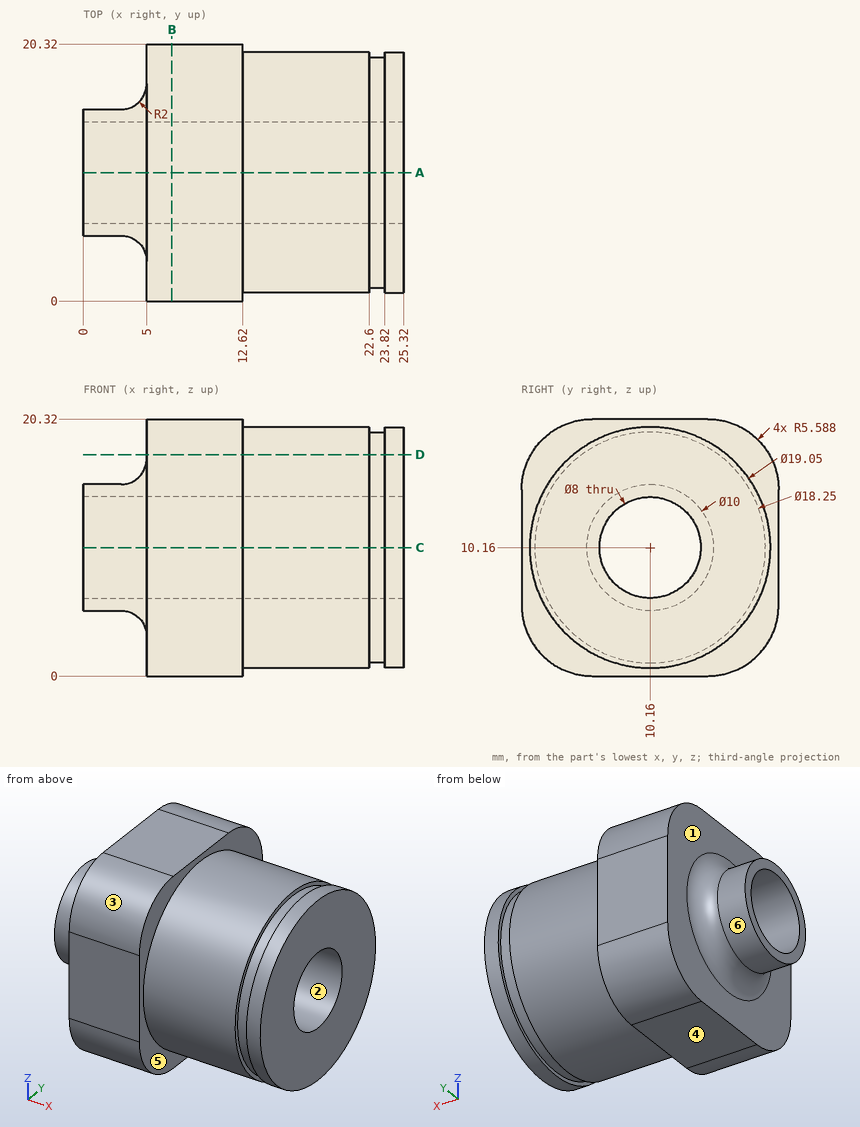
The drawing under review shows one solid part. Ordinate dimensions are in mm from its lowest x, y, z. A direction names the side the tool comes from. Coordinates: 2 decimals unless noted, no trailing zeros. Loops run counter-clockwise (first coordinate to the right, second up) from the corner with the lowest first, then second, coordinate; pieces in that order, holes last. Notation, with made-up numbers: (85.5, 39) - (97.5, 39) arc R27 ccw to (97.5, 65) - close; hole circle Ø5 at (27, -36.5). An arc over 180 degrees is marked (long way). Return JSON: item names as keys, results as strings.
Item 1: Take a section at B-B (x = 7). Give the boundary of the cut face in (y, z), then the cut area to 3 significant figures.
Determined:
{"outline": "(0, 5.59) arc R5.59 ccw to (5.59, 0) - (14.73, 0) arc R5.59 ccw to (20.32, 5.59) - (20.32, 14.73) arc R5.59 ccw to (14.73, 20.32) - (5.59, 20.32) arc R5.59 ccw to (0, 14.73) - close; hole circle Ø8 at (10.16, 10.16)", "area": "336 mm2"}
Item 2: For the marked faces 4, 5 and 6, list the 3-axis set-ups (+Z, -Z, +X, -X, +Y, -Y) from which the entire face can be reached by the end or side of a thin tool; tool diameter is ignored.
Determined:
{"face 4": "-Z, +X, -X, +Y, -Y", "face 5": "+X", "face 6": "-X"}
Item 3: Take a section at D-D (z = 17.5). Give the boundary of the cut face in (x, y), then the cut area to 3 significant figures.
Determined:
{"outline": "(5, 0.73) - (12.62, 0.73) - (12.62, 4.09) - (22.6, 4.09) - (22.6, 4.74) - (23.82, 4.74) - (23.82, 4.09) - (25.32, 4.09) - (25.32, 16.23) - (23.82, 16.23) - (23.82, 15.58) - (22.6, 15.58) - (22.6, 16.23) - (12.62, 16.23) - (12.62, 19.59) - (5, 19.59) - close", "area": "296 mm2"}
Item 4: For line 1 (Y direction, x = 15.5, z = 10.16) (3 decimals); line 2 (X direction, y = 1, z = 11.25); line 3 (Y direction, x = 9.5, z = 10.16), list the stretches that pass through material, from the lowest coordinate up.
Determined:
{"line 1": "y = 0.635 to 6.16, 14.16 to 19.685", "line 2": "x = 5 to 22.6, 23.82 to 25.32", "line 3": "y = 0 to 6.16, 14.16 to 20.32"}
Item 5: Mouldability with a two-part tool opening along Y and no side actions: class the marked faces 1, 2 and 3 as pulls with the +Y half, pulls with the -Y half, needs draft (parallel to the pull), parting line crosses it, or undercut.
Determined:
{"face 1": "needs draft", "face 2": "undercut", "face 3": "pulls with the -Y half"}
Item 6: Insertion check: pin 1 (1.5 mm diameter, centred on x = 13.5, y = 9.5, fed in from +Z) (3 decimals); pin 2 (1.5 mm diameter, centred on x = 14, y = 10.5, fed in from -Z) (3 decimals); pin 3 (6 mm diameter, centred on x = 18, y = 4.5, fed in from -Z). Each pin has a flat end and moves straight along its axis. Give the tip position at first contact, or say it passes through.
Determined:
{"pin 1": "stops at z = 19.685", "pin 2": "stops at z = 0.635", "pin 3": "stops at z = 1.01"}
Item 7: Take a section at A-A (y = 10.16). Give the boundary of the cut face in (x, z) (3 decimals).
Determined:
{"outline": "(0, 5.16) - (3, 5.16) arc R2 cw to (5, 3.16) - (5, 0) - (12.62, 0) - (12.62, 0.635) - (22.6, 0.635) - (22.6, 1.035) - (23.82, 1.035) - (23.82, 0.635) - (25.32, 0.635) - (25.32, 6.16) - (0, 6.16) - close; (0, 14.16) - (25.32, 14.16) - (25.32, 19.685) - (23.82, 19.685) - (23.82, 19.285) - (22.6, 19.285) - (22.6, 19.685) - (12.62, 19.685) - (12.62, 20.32) - (5, 20.32) - (5, 17.16) arc R2 cw to (3, 15.16) - (0, 15.16) - close"}
